Can you work these out from the model? Positions are in its coordinate system, mm. Coordinates: 2 decimals unless noted, no trailing zeros. Write each loop counter-clockwise with the first axis right and the second up, starting at its lowest first coordinate (ties: lowest second). Pieces come first, ordered by that corner, then holes.
```python
from build123d import *

# Parameters (mm, degrees)
TRUNCATED_BALL_DEPTH      = 13.7
TRUNCATED_BALL_DEPTH_BACK = 13.7
SKETCH3_R                 = 8.4582
RECESSED_DEPTH            = 0.127
SKETCH4_R                 = 2.54
THREADED_DEPTH            = 6.35
CHAMFER2_SIZE             = 0.635


with BuildPart() as part:
    # Sketch1 → Complete_Ball (revolve)
    with BuildSketch(Plane.XY):
        with BuildLine():
            Line((0, 12.7), (0, -12.7))
            ThreePointArc((0, -12.7), (12.7, 0), (0, 12.7))
        make_face()
    revolve(axis=Axis((0, 13.6525, 0), (0, -1, 0)))

    # Sketch2 → Truncated_ball (cut, two sides)
    with BuildSketch(Plane.XY) as truncated_ball_sk:
        with BuildLine():
            Line((-10.998522628, -6.35), (10.998522628, -6.35))
            ThreePointArc((10.998522628, -6.35), (0, -12.7), (-10.998522628, -6.35))
        make_face()
    extrude(amount=TRUNCATED_BALL_DEPTH, mode=Mode.SUBTRACT)
    extrude(truncated_ball_sk.sketch, amount=-TRUNCATED_BALL_DEPTH_BACK, mode=Mode.SUBTRACT)

    # Sketch3 → Recessed (cut)
    with BuildSketch(Plane.XZ.offset(6.35)):
        with Locations(Location((0, 0, 0), (0, 0, 270))):  # turned: the seam where the file's is
            Circle(SKETCH3_R)
    extrude(amount=-RECESSED_DEPTH, mode=Mode.SUBTRACT)

    # Sketch4 → Threaded (cut)
    with BuildSketch(Plane.XZ.offset(6.223)):
        with Locations(Location((0, 0, 0), (0, 0, 270))):  # turned: the seam where the file's is
            Circle(SKETCH4_R)
    extrude(amount=-THREADED_DEPTH, mode=Mode.SUBTRACT)

    # Chamfer2
    chamfer2_edges = [part.edges().sort_by_distance(p)[0] for p in [
        (0, -6.223, 2.54),
    ]]
    chamfer(chamfer2_edges, length=CHAMFER2_SIZE)


solid = part.part
```
1. I'm going to push flat-ended pins straight in: P1, Ø8, axis at x = 9.5, y = -0.5, coming from the +Z side; P2, Ø6, axis at y = 7.5, z = 7.5, coming from the +X side; P3, Ø1, axis at y = 4, z = 6.5, coming from the -X side; P4, Ø8, axis at x = -10, z = 10, coming from the -Y side. Where does each tip first touch, or does it pass through?
2. If I drill on L1, parallel to X at y = -4.35, z = 0; L2, parallel to Y at x = -1.75, z = -0.5; L3, parallel to X at y = 6.75, z = 0.5, over which ranges is the centre line in solid material (lowest first)?
3. If we section it at C-C, the plane z = 5.75: List the corners of the cut face in (x, y) for me.
4. If we section it at A-A, the plane x = 0: List the corners of the cut face in (y, z) for me (3 decimals).
5. We'd pull the mould along Z, two halves only. Please class faces 1 (the face through (2.52, -2.77, 0.33)), 2 (the face through (5.7, -6.35, 6.5)): released by +Z, released by -Z, zero draft, split by the parting line, or undercut.
6. If we section it at B-B, the plane z = 0: List the corners of the cut face in (x, y) for me (3 decimals), plus the area to 3 significant figures.
7. If we section it at D-D, the plane x = 7.5: List the corners of the cut face in (y, z) for me, plus the area to 3 significant figures.
Answers:
1. P1: stops at z = 11.44
1. P2: stops at x = 10.17
1. P3: stops at x = -10.51
1. P4: stops at y = -6.35
2. L1: x = -11.93 to -2.54, 2.54 to 11.93
2. L2: y = 0.13 to 12.57
2. L3: x = -10.75 to 10.75
3. outline: (-9.38, -6.35) - (-6.2, -6.35) - (-6.2, -6.22) - (6.2, -6.22) - (6.2, -6.35) - (9.38, -6.35) arc R11.32 ccw (long way) to start
4. outline: (-6.35, -10.999) arc R12.7 ccw (long way) to (-6.35, 10.999) - (-6.35, 8.458) - (-6.223, 8.458) - (-6.223, 3.175) - (-5.588, 2.54) - (0.127, 2.54) - (0.127, -2.54) - (-5.588, -2.54) - (-6.223, -3.175) - (-6.223, -8.458) - (-6.35, -8.458) - close
5. face 1: undercut
5. face 2: zero draft
6. outline: (-10.999, -6.35) - (-8.458, -6.35) - (-8.458, -6.223) - (-3.175, -6.223) - (-2.54, -5.588) - (-2.54, 0.127) - (2.54, 0.127) - (2.54, -5.588) - (3.175, -6.223) - (8.458, -6.223) - (8.458, -6.35) - (10.999, -6.35) arc R12.7 ccw (long way) to start
6. area: 373 mm2
7. outline: (-6.35, -8.04) arc R10.25 ccw (long way) to (-6.35, 8.04) - (-6.35, 3.91) - (-6.22, 3.91) - (-6.22, -3.91) - (-6.35, -3.91) - close
7. area: 285 mm2
